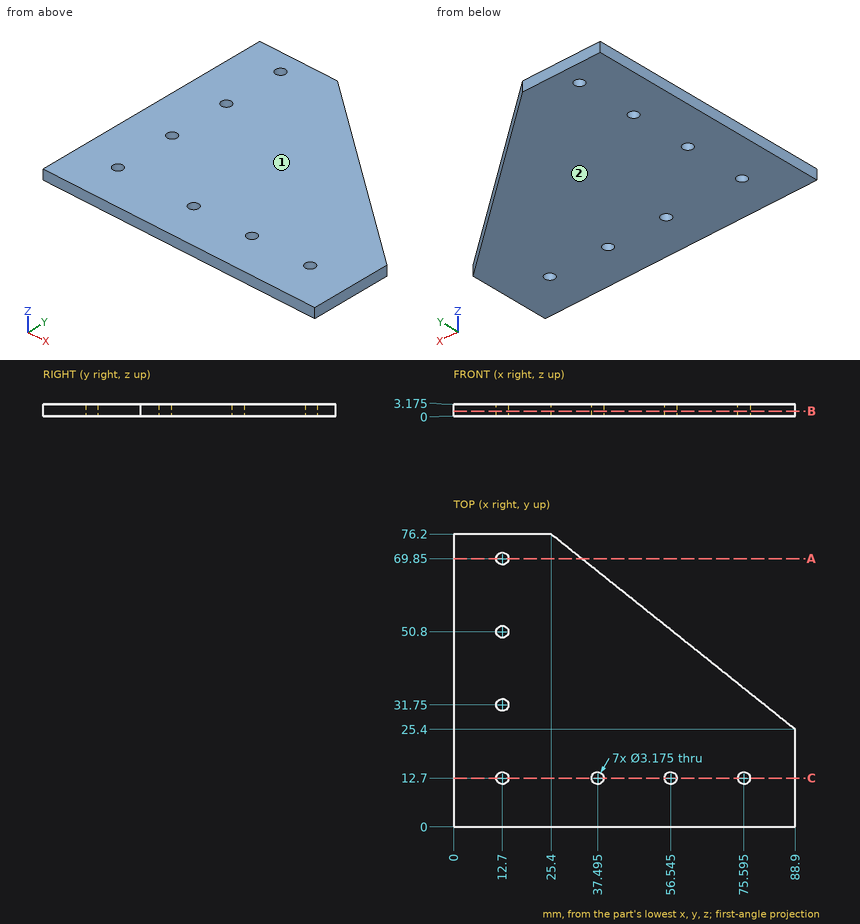
Job drawing, mm, ordinate dimensions from the low corner. One solid piece. Coordinates: 2 decimals unless noted, no trailing zeros. Order: outer loops, then holes, each group sorted by start corner. A loop starts at its lowest first (then second) coordinate and runs counter-clockwise, first axis right, second up. Notation, with made-up numbers: (-32.5, 30.5) - (16.5, 30.5) arc R22 cw to (16.5, 59.5) - close; hole circle Ø8 at (53, 63.25). An arc over 180 degrees is marked (long way). Write each question's results on one line, items separated by ' | '. Start each with the question number.
Item 1: Band-saw the part on A-A on y = 69.85. Write the cut outline in (x, z) (1 decimal).
Item 2: Band-saw the part on B-B on z = 1.3. State how many separate pieces and enclosed holes the cut face has, and give its area (3 significant figures).
Item 3: Flat gauge pin, fed straight in: pin 1 (12 mm diameter, centred on x = 71, y = 41, fed in from +Z) (3 decimals). Where does the tip first touch, or does it go through?
Item 4: Mould opens along Z. For the marked faces 1 and 2 say: released by +Z, released by -Z, zero draft, split by the parting line, or undercut.
Item 5: Wall check: probe 1 along Y at (x, z) = (12.7, 0.8); probe 2 along X at (y, z) = (69.85, 0.75); probe 3 along X at (y, z) = (49.5, 1.9) (1 decimal). Give the ranges that are in metal, low to high. Write a range as [from, to].
Item 6: Band-saw the part on C-C on y = 12.7. Write the cut outline in (x, z) (1 decimal).
Numbers:
1) outline: (0, 0) - (11.1, 0) - (11.1, 3.2) - (0, 3.2) - close; (14.3, 0) - (33.3, 0) - (33.3, 3.2) - (14.3, 3.2) - close
2) separate pieces: 1 | enclosed holes: 7 | area: 5,110 mm^2
3) pin 1: z = 3.175
4) face 1: released by +Z | face 2: released by -Z
5) probe 1: [0, 11.11], [14.29, 30.16], [33.34, 49.21], [52.39, 68.26], [71.44, 76.2] | probe 2: [0, 11.11], [14.29, 33.34] | probe 3: [0, 11.8], [13.6, 58.8]
6) outline: (0, 0) - (11.1, 0) - (11.1, 3.2) - (0, 3.2) - close; (14.3, 0) - (35.9, 0) - (35.9, 3.2) - (14.3, 3.2) - close; (39.1, 0) - (55, 0) - (55, 3.2) - (39.1, 3.2) - close; (58.1, 0) - (74, 0) - (74, 3.2) - (58.1, 3.2) - close; (77.2, 0) - (88.9, 0) - (88.9, 3.2) - (77.2, 3.2) - close
